from build123d import *

# Parameters (mm, degrees)
SKETCH1_R           = 81
SKETCH1_R_2         = 22.225
SKETCH1_R_3         = 4
BOSS_EXTRUDE1_DEPTH = 14.5
SKETCH2_R           = 87.498812031
SKETCH2_R_2         = 64.75
CUT_EXTRUDE1_DEPTH  = 3


with BuildPart() as part:
    # Sketch1 → Boss-Extrude1 (new body)
    with BuildSketch(Plane(origin=(0, 0, 0), x_dir=(1, 0, 0), z_dir=(0, 1, 0))):
        with Locations(Location((0, 0, 0), (0, 0, 270))):
            Circle(SKETCH1_R)
        with Locations(Location((0, 0, 0), (0, 0, 270))):
            Circle(SKETCH1_R_2, mode=Mode.SUBTRACT)
        with Locations(Location((0, 71, 0), (0, 0, 270))):
            Circle(SKETCH1_R_3, mode=Mode.SUBTRACT)
        with Locations(Location((61.487803669, 35.5, 0), (0, 0, 270))):
            Circle(SKETCH1_R_3, mode=Mode.SUBTRACT)
        with Locations(Location((61.487803669, -35.5, 0), (0, 0, 270))):
            Circle(SKETCH1_R_3, mode=Mode.SUBTRACT)
        with Locations(Location((0, -71, 0), (0, 0, 270))):
            Circle(SKETCH1_R_3, mode=Mode.SUBTRACT)
        with Locations(Location((-61.487803669, -35.5, 0), (0, 0, 270))):
            Circle(SKETCH1_R_3, mode=Mode.SUBTRACT)
        with Locations(Location((-61.487803669, 35.5, 0), (0, 0, 270))):
            Circle(SKETCH1_R_3, mode=Mode.SUBTRACT)
    extrude(amount=-BOSS_EXTRUDE1_DEPTH)

    # Sketch2 → Cut-Extrude1 (cut)
    with BuildSketch(Plane(origin=(0, 0, 0), x_dir=(1, 0, 0), z_dir=(0, 1, 0))):
        Circle(SKETCH2_R)
        with Locations(Location((0, 0, 0), (0, 0, 270))):
            Circle(SKETCH2_R_2, mode=Mode.SUBTRACT)
    extrude(amount=-CUT_EXTRUDE1_DEPTH, mode=Mode.SUBTRACT)


solid = part.part
Input: part model. Units: mm. Frame: model coordinates. A direction names the side the tool comes from. Coordinates: 2 decimals unless noted, no trailing zeros. Write each loop counter-clockwise with the first axis right and the second up, starting at its lowest first coordinate (ties: lowest second). Pieces come first, ordered by that corner, then holes. Notation, with made-up numbers: M 5.5,-34.5 L 62.5,-34.5 A25 ccw 62.5,-5.5 Z; hole C -1,-12 d3. An arc over 180 degrees is marked long. Answer as a JSON object with one key per item and string values. Group by question number.
(1) Section D-D on z = 2. Output: boundary loops of the cut face in (x, y), plus the area to 3 significant figures.
(2) Mould query, pull axis X, two halves, no side actions, for faces 1 (the face through (-17, -14.5, 17)), 2 (the face through (68.3, -8.67, 43.545)), 3 (the face through (65.454, -8.67, -36.021)). Classes: pulls with the +X half, pulls with the -X half, needs draft (parallel to the pull), parting line crosses it, or undercut.
(3) Section A-A on x = 0. Output: boundary loops of the cut face in (y, z) (3 decimals), plus the area to 3 significant figures.
(4) Section C-C on x = -16.5. Output: boundary loops of the cut face in (y, z), plus the area to 3 significant figures.
(5) Ray query, line 1 along X through (y, z) = (-11.25, -35.5); line 2 along X through (y, z) = (-9.5, 0) (3 decimals); line 3 along X through (y, z) = (-4.75, -36). Return the intervals inside material, ascending. Write a range as [from, to].
(6) Contact query for flat-ended pins moving along their axis: P1, Ø3, axis at x = 64.5, y = -9.5, coming from the +Z side; P2, Ø6, axis at x = 16.5, y = -7.5, coming from the +Z side; P3, Ø9, axis at x = 61.49, z = -35.5, coming from the +Y side. Output: stop coordinate, or through.
(7) Section B-B on z = -35.5. Output: boundary loops of the cut face in (x, y).
(8) Set-up query: faces 4 (the face through (-24.4, -3, -60.4)), 5 (the face through (18.74, -7.15, 11.95)). Return all of +Z, -Z, +X, -X, +Y, -Y with unobstructed straight access to the full face (end or side cutting, diameter ignored); none if empty.
Result set:
{
 "1": {"outline": "M -80.98,-14.5 L -22.13,-14.5 L -22.13,0 L -64.72,0 L -64.72,-3 L -80.98,-3 Z; M 22.13,-14.5 L 80.98,-14.5 L 80.98,-3 L 64.72,-3 L 64.72,0 L 22.13,0 Z", "area": "1,610 mm2"},
 "2": {"face 1": "needs draft", "face 2": "parting line crosses it", "face 3": "undercut"},
 "3": {"outline": "M -14.5,-81 L -3,-81 L -3,-75 L -14.5,-75 Z; M -14.5,-67 L -3,-67 L -3,-64.75 L 0,-64.75 L 0,-22.225 L -14.5,-22.225 Z; M -14.5,22.225 L 0,22.225 L 0,64.75 L -3,64.75 L -3,67 L -14.5,67 Z; M -14.5,75 L -3,75 L -3,81 L -14.5,81 Z", "area": "1,420 mm2"},
 "4": {"outline": "M -14.5,-79.3 L -3,-79.3 L -3,-62.61 L 0,-62.61 L 0,-14.89 L -14.5,-14.89 Z; M -14.5,14.89 L 0,14.89 L 0,62.61 L -3,62.61 L -3,79.3 L -14.5,79.3 Z", "area": "1,770 mm2"},
 "5": {"line 1": "x = [-72.81, -65.49], [-57.49, 57.49], [65.49, 72.81]", "line 2": "x = [-81, -22.225], [22.225, 81]", "line 3": "x = [-72.56, -65.46], [-57.52, 57.52], [65.46, 72.56]"},
 "6": {"P1": "stops at z = 50.91", "P2": "stops at z = 79.87", "P3": "stops at y = -3"},
 "7": {"outline": "M -72.81,-14.5 L -65.49,-14.5 L -65.49,-3 L -72.81,-3 Z; M -57.49,-14.5 L 57.49,-14.5 L 57.49,-3 L 54.15,-3 L 54.15,0 L -54.15,0 L -54.15,-3 L -57.49,-3 Z; M 65.49,-14.5 L 72.81,-14.5 L 72.81,-3 L 65.49,-3 Z"},
 "8": {"face 4": "+Y", "face 5": "+Y, -Y"}
}
